Here's how the part is built. I have some questions about the finished solid (model axes, mm). Face numbers are marked on the shaded views. A direction names the side the tool comes from. Coordinates: 2 decimals unless noted, no trailing zeros. Write each loop counter-clockwise with the first axis right and the second up, starting at its lowest first coordinate (ties: lowest second). Pieces come first, ordered by that corner, then holes. Notation, with made-up numbers: (6.25, 13.5) -> (34.25, 13.5) arc R19 cw to (34.25, 29.5) -> close; hole circle Ø4 at (0.25, 39.5). An arc over 180 degrees is marked (long way). Use a Markdown table: item, result. Add a question column.
Item 1: If we mould it in two halves opening along X, with no side actions, what happens to the marked faces 5, 6 and 7? For each: pulls with the +X half, pulls with the -X half, needs draft (parallel to the pull), parting line crosses it, or undercut.
Item 2: If I drill on line 1 along Z through (x, y) = (4.5, 2); line 2 along Y through (x, z) = (0, 3.5), over which ranges is the centre line in solid material (lowest first)? Write a range as from..to.
Item 3: On a 3-axis mill with a long thin cutter (end or side, diameter ignored), from which of +Z, -Z, +X, -X, +Y, -Y can I reach the whole of each face in a straight line? I mean the marked faces 1, 2, 3 and 4. Say none if no direction works.
Item 4: Will these pins go through, and if not, where does the flat tip stop? pin 1 Ø1.5 at (y, z) = (2.5, 4.5) entering from -X; pin 2 Ø1.5 at (y, z) = (-5, 5.5) entering from -X.
Item 5: Imagine slicing it at D-D, the plane z = 5.75. Write out the boundary of the cut face in (x, y).
Item 6: Imagine slicing it at A-A, the plane x = 0. Write out the boundary of the cut face in (y, z).
Autodesk Inventor part; units mm, degrees
ref_plane "YZ Plane" through (0, 0, 0) normal (1, 0, 0) x (0, 1, 0)
ref_plane "XZ Plane" through (0, 0, 0) normal (0, 1, 0) x (-1, 0, 0)
ref_plane "XY Plane" through (0, 0, 0) normal (0, 0, 1) x (1, 0, 0)
sketch "Sketch1" plane through (0, 0, 0) normal (0, 0, 1) x (1, 0, 0)
  circle A0 centre (0, 0) radius 6.3
  dimension "d0" = 12.6
extrude "Extrusion1" add sketch "Sketch1" along normal blind 1
sketch "Sketch2" plane through (0, 0, 1) normal (0, 0, 1) x (1, 0, 0)
  circle A0 centre (0, 0) radius 6.3
  circle A1 centre (0, 0) radius 4.75
  dimension "d3" = 9.5
extrude "Extrusion2" add sketch "Sketch2" along normal blind 4.5 contours A1
sketch "Sketch3" plane through (0, 0, 5.5) normal (0, 0, 1) x (1, 0, 0)
  circle A0 centre (0, 0) radius 4.75
  circle A1 centre (0, 4.75) radius 0.65
  dimension "d6" = 1.3
extrude "Extrusion3" cut sketch "Sketch3" against normal blind 4.5 contours A1 A0 | A0 A1 picked at (-0.025, 4.5315) picked at (0.0193, 4.9625)
pattern_circular "Circular Pattern1" count 16 over 360 about axis through (0, 0, 1) along (0, 0, 1) of "Extrusion3"
sketch "Sketch4" plane through (0, 0, 5.5) normal (0, 0, 1) x (1, 0, 0)
  arc A0 (2.8688, 3.7859) -> (2.3998, 4.0992) centre (0, 0) ccw
  circle A1 centre (0, 0) radius 6.3
  dimension "d12" = 12.6
extrude "Extrusion4" add sketch "Sketch4" along normal blind 1
sketch "Sketch5" plane through (0, 0, 6.5) normal (0, 0, 1) x (1, 0, 0)
  circle A0 centre (0, 0) radius 6.3
hole "Hole1" at (0, 0, 6.5) direction (0, 0, -1) diameter 5 end through all
chamfer "Chamfer1" distance 0.5 angle 45 2 edges at (-6.3, 0, 5.5) (-6.3, 0, 1)
properties part number "stepper_gear_28"
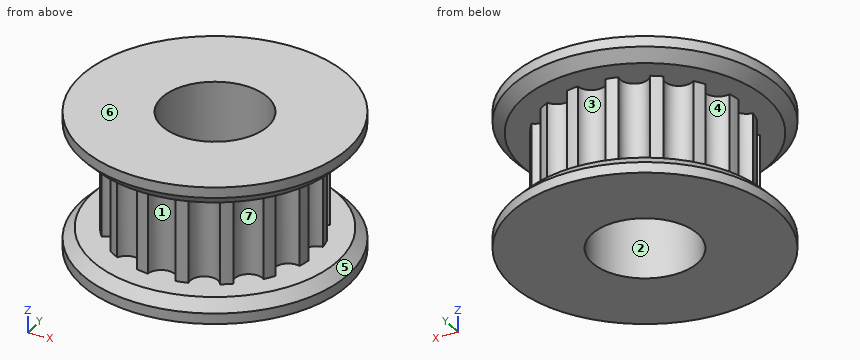
Ans:
| question | item | result |
|---|---|---|
| 1 | face 5 | parting line crosses it |
| 1 | face 6 | needs draft |
| 1 | face 7 | undercut |
| 2 | line 1 | z = 0..1, 5.5..6.5 |
| 2 | line 2 | y = -4.1..-2.5, 2.5..4.1 |
| 3 | face 1 | -Y |
| 3 | face 2 | +Z, -Z |
| 3 | face 3 | +Y |
| 3 | face 4 | none |
| 4 | pin 1 | stops at x = -4.1 |
| 4 | pin 2 | stops at x = -4.47 |
| 5 | outline | circle Ø12.1 at (0, 0); hole circle Ø5 at (0, 0) |
| 6 | outline | (-6.3, 0) -> (-2.5, 0) -> (-2.5, 6.5) -> (-6.3, 6.5) -> (-6.3, 6) -> (-5.8, 5.5) -> (-4.1, 5.5) -> (-4.1, 1) -> (-5.8, 1) -> (-6.3, 0.5) -> close; (2.5, 0) -> (6.3, 0) -> (6.3, 0.5) -> (5.8, 1) -> (4.1, 1) -> (4.1, 5.5) -> (5.8, 5.5) -> (6.3, 6) -> (6.3, 6.5) -> (2.5, 6.5) -> close |
